Could you check a few things on this model? Use its own coordinates, in mm. Coordinates: 2 decimals unless noted, no trailing zeros. Order: outer loops, then holes, each group sorted by start corner. A loop starts at its lowest first (then second) coordinate and runs counter-clockwise, first axis right, second up. Notation, with made-up numbers: (18.5, 24.25) -> (30.5, 24.25) arc R16 cw to (30.5, 45.25) -> close; hole circle Ø2 at (82, -22.5). An arc over 180 degrees is marked (long way). Use a Markdown table: item, result. Add a question column.
1) If we section it at A-A (z = 0): Write out the boundary of the cut face in (x, y).
2) If we section it at B-B (x = 0): Write out the boundary of the cut face in (y, z).
3) If we section it at D-D (y = 11): Write out the boundary of the cut face in (x, z), plus the area to 3 significant figures.
4) If we section it at C-C (x = -10): Write out the boundary of the cut face in (y, z).
5) Thinking about a two-plate mould opening in Z: for faces 1 (the cylindrical face through (-10.464, 12.535, -0.325)), 2 (the cylindrical face through (-1.532, 4.93, 3.695)), 3 (the cylindrical face through (10.464, 12.535, 0.325)), 4 (the flat face through (3, 10, -3)), which applies, +Z half, -Z half, draft (parallel to the pull), parting line (faces both ways), or undercut?
6) If I drill on L1, parallel to X at y = 13, z = 0; L2, parallel to Z at x = -1, y = 12.75; L3, parallel to X at y = 7.75, z = 0, over which ranges is the centre line in solid material (lowest first)? Write a range as [from, to].
7) Will these pins go through, and if not, where does the flat tip stop? pin 1 Ø4 at (x, y) = (0, 4) entering from -Z; pin 2 Ø8 at (x, y) = (-2.5, 2.5) entering from +Z; pin 3 Ø3 at (x, y) = (2.5, 2.5) entering from -Z; pin 4 Ø2.5 at (x, z) = (0, -9) entering from +Y (3 decimals).
```python
from build123d import *

# Parameters (mm, degrees)
SKETCH1_R                = 4
BOSS_EXTRUDE1_DEPTH      = 10
SKETCH3_R                = 12.5
BOSS_EXTRUDE2_DEPTH      = 5
F_3_0_3_DIAMETER_HOLE2_D = 3
SKETCH6_R                = 1.5
CUT_EXTRUDE2_DEPTH       = 10
SKETCH2_R                = 2
CUT_EXTRUDE1_DEPTH       = 24.184046239
CIRPATTERN1_COUNT        = 4


with BuildPart() as part:
    # Sketch1 → Boss-Extrude1 (new body)
    with BuildSketch(Plane(origin=(0, 0, 0), x_dir=(1, 0, 0), z_dir=(0, 1, 0))):
        with Locations(Location((0, 0, 0), (0, 0, 270))):
            Circle(SKETCH1_R)
    extrude(amount=BOSS_EXTRUDE1_DEPTH)

    # Sketch3 → Boss-Extrude2 (add)
    with BuildSketch(Plane(origin=(0, 10, 0), x_dir=(1, 0, 0), z_dir=(0, 1, 0))):
        with Locations(Location((0, 0, 0), (0, 0, 270))):
            Circle(SKETCH3_R)
    extrude(amount=BOSS_EXTRUDE2_DEPTH)

    # Ø3.0 (3) Diameter Hole2 (through all)
    with Locations(Plane(origin=(0, 4, -4), x_dir=(-1, 0, 0), z_dir=(0, 0, -1))):
        with Locations((0, 0)):
            Hole(F_3_0_3_DIAMETER_HOLE2_D / 2)

    # Sketch6 → Cut-Extrude2 (cut)
    with BuildSketch(Plane(origin=(0, 15, 0), x_dir=(1, 0, 0), z_dir=(0, 1, 0))):
        with Locations(Location((-9, 0, 0), (0, 0, 270))):
            Circle(SKETCH6_R)
    cut_extrude2 = extrude(amount=-CUT_EXTRUDE2_DEPTH, mode=Mode.SUBTRACT)

    # Sketch2 → Cut-Extrude1 (cut, through all)
    with BuildSketch(Plane.XZ):
        with Locations(Location((0, 0, 0), (0, 0, 270))):
            Circle(SKETCH2_R)
    extrude(amount=-CUT_EXTRUDE1_DEPTH, mode=Mode.SUBTRACT)

    # CirPattern1: Cut-Extrude2 ×4 about axis
    cirpattern1_axis = Axis((0, 0, 0), (0, 1, 0))
    for i in range(1, CIRPATTERN1_COUNT):
        add(cut_extrude2.rotate(cirpattern1_axis, i * 360 / CIRPATTERN1_COUNT), mode=Mode.SUBTRACT)


solid = part.part
```
Answer sheet:
| question | item | result |
|---|---|---|
| 1 | outline | (-12.5, 10) -> (-10.5, 10) -> (-10.5, 15) -> (-12.5, 15) -> close; (-7.5, 10) -> (-4, 10) -> (-4, 0) -> (-2, 0) -> (-2, 15) -> (-7.5, 15) -> close; (2, 0) -> (4, 0) -> (4, 10) -> (7.5, 10) -> (7.5, 15) -> (2, 15) -> close; (10.5, 10) -> (12.5, 10) -> (12.5, 15) -> (10.5, 15) -> close |
| 2 | outline | (0, -4) -> (2.5, -4) -> (2.5, -2) -> (0, -2) -> close; (0, 2) -> (2.5, 2) -> (2.5, 4) -> (0, 4) -> close; (5.5, -4) -> (10, -4) -> (10, -7.5) -> (15, -7.5) -> (15, -2) -> (5.5, -2) -> close; (5.5, 2) -> (15, 2) -> (15, 7.5) -> (10, 7.5) -> (10, 4) -> (5.5, 4) -> close; (10, -12.5) -> (15, -12.5) -> (15, -10.5) -> (10, -10.5) -> close; (10, 10.5) -> (15, 10.5) -> (15, 12.5) -> (10, 12.5) -> close |
| 3 | outline | circle Ø25 at (0, 0); hole circle Ø3 at (-9, 0); hole circle Ø4 at (0, 0); hole circle Ø3 at (0, -9); hole circle Ø3 at (0, 9); hole circle Ø3 at (9, 0) |
| 3 | area | 450 mm2 |
| 4 | outline | (10, -7.5) -> (15, -7.5) -> (15, -1.12) -> (10, -1.12) -> close; (10, 1.12) -> (15, 1.12) -> (15, 7.5) -> (10, 7.5) -> close |
| 5 | face 1 | undercut |
| 5 | face 2 | parting line |
| 5 | face 3 | undercut |
| 5 | face 4 | draft |
| 6 | L1 | [-12.5, -10.5], [-7.5, -2], [2, 7.5], [10.5, 12.5] |
| 6 | L2 | [-12.46, -10.12], [-7.88, -1.73], [1.73, 7.88], [10.12, 12.46] |
| 6 | L3 | [-4, -2], [2, 4] |
| 7 | pin 1 | z = -4 |
| 7 | pin 2 | z = 4 |
| 7 | pin 3 | z = -3.87 |
| 7 | pin 4 | through |
